Source: CAD feature listing. Evaluate the final solid. Frame: model axes, mm. A direction names the side the tool comes from. Give positions to 0.01 mm unless a question says otherwise; leave off trailing zeros. Order: outer loops, then holes, each group sorted by start corner. A loop starts at its lowest first (then second) coordinate and runs counter-clockwise, first axis right, second up. Notation, with made-up numbers: (-13, 39.5) - (6, 39.5) arc R20 ccw to (6, 77.5) - close; hole circle Ø3 at (35.25, 34.5). An arc over 180 degrees is marked (long way). Answer as CSV lines item,"result".
Autodesk Inventor part; units mm, degrees
ref_plane "YZ Plane" through (0, 0, 0) normal (1, 0, 0) x (0, 1, 0)
ref_plane "XZ Plane" through (0, 0, 0) normal (0, 1, 0) x (-1, 0, 0)
ref_plane "XY Plane" through (0, 0, 0) normal (0, 0, 1) x (1, 0, 0)
sketch "Skizze1" plane through (0, 0, 0) normal (0, 0, 1) x (1, 0, 0)
  line L0 (-5.275, 5.275) -> (5.275, 5.275)
  line L1 (5.275, 5.275) -> (5.275, -5.275)
  line L2 (5.275, -5.275) -> (-5.275, -5.275)
  line L3 (-5.275, -5.275) -> (-5.275, 5.275)
  line L4 (-5.275, 5.275) -> (5.275, -5.275) construction
  line L5 (5.275, 5.275) -> (-5.275, -5.275) construction
  line L6 (8.275, 8.275) -> (-8.275, 8.275)
  line L7 (-8.275, 8.275) -> (-8.275, -8.275)
  line L8 (-8.275, -8.275) -> (8.275, -8.275)
  line L9 (8.275, -8.275) -> (8.275, 8.275)
  point P0 (0, 0)
  dimension "d0" = 10.55
  dimension "d1" = 10.55
  dimension "d2" = 3
extrude "Extrusion1" add sketch "Skizze1" along normal blind 15
sketch "Skizze2" plane through (8.275, -8.275, 0) normal (1, 0, 0) x (0, 0, -1)
  line L0 (0, 0) -> (0, 16.55)
  line L1 (0, 16.55) -> (-15, 16.55)
  line L2 (-15, 0) -> (-15, 16.55)
  line L3 (0, 0) -> (-15, 0)
  circle A0 centre (-7.5, 22) radius 2.1
  circle A1 centre (-7.5, 22) radius 5.3
  line L4 (-15, 16.55) -> (-12.8, 22)
  line L5 (0, 16.55) -> (0, 0)
  line L6 (0, 16.55) -> (-2.2, 22)
  point P0 (0, 8.275)
  dimension "d5" = 4.2
  dimension "d6" = 22
  dimension "d7" = 7.5
  dimension "d8" = 3.2
extrude "Extrusion2" add sketch "Skizze2" against normal up to surface (16.55 mm away) contours L1 L4 A1 L6 | A1
fillet "Rundung1" radius 15.75 4 edges at (0, 13.725, 2.2) (0, 8.275, 0) (0, 8.275, 15) (0, 13.725, 12.8)
equation "\"d1\" = d0"
properties part number "AL_PipeMount"
(1) Access query for faces 1 (the flat face through (-5.275, 0, 7)), 2 (the cylindrical face through (0.116, 13.251, 13.067)). Directions: +Z, -Z, +X, -X, +Y, -Y. A direction counts if a zero-diameter tool reaches every point of the face in a straight line with its end or side. Return the directions, or none.
Completed:
face 1,"+Z, -Z"
face 2,"+Z, +X, -X, +Y"
(2) Mould query, pull axis X, two halves, no side actions, for faces 3 (the cylindrical face through (0.1, 13.8, 9.6)), 4 (the flat face through (5.275, 0, 7)), 5 (the flat face through (8.275, 2, 7)). Classes: released by +X, released by -X, zero draft, split by the parting line, or undercut.
Completed:
face 3,"zero draft"
face 4,"undercut"
face 5,"released by +X"
(3) Cut plane D-D (z = 12.25). Return loops of the section in (x, y) (3 decimals), then the cut area to 3 significant figures.
Completed:
outline,"(-8.275, -8.275) - (8.275, -8.275) - (8.275, 16.076) - (-8.275, 16.076) - close; hole (-5.275, -5.275) - (5.275, -5.275) - (5.275, 5.275) - (-5.275, 5.275) - close"
area,"292 mm²"
(4) Cut plane A-A (z = 7.5). Return loops of the section in (x, y) (3 decimals), then the cut area to 3 significant figures.
Completed:
outline,"(-8.275, -8.275) - (8.275, -8.275) - (8.275, 11.625) - (-8.275, 11.625) - close; (-8.275, 15.825) - (8.275, 15.825) - (8.275, 19.025) - (-8.275, 19.025) - close; hole (-5.275, -5.275) - (5.275, -5.275) - (5.275, 5.275) - (-5.275, 5.275) - close"
area,"271 mm²"
(5) Ray query, line 1 (Y direction, x = -0.25, z = 7.5) (3 decimals); line 2 (X direction, y = 3.75, z = 13.75) (3 decimals); line 3 (Z direction, x = -3.5, y = 11). Return the intervals inside material, ascending. Write a range as from..to.
Completed:
line 1,"-8.275..-5.275, 5.275..11.625, 15.825..19.025"
line 2,"-8.275..-5.275, 5.275..8.275"
line 3,"1.1..13.9"
(6) Cut plane C-C (x = 0). Return loops of the section in (y, z) (3 decimals).
Completed:
outline,"(-8.275, 0) - (-5.275, 0) - (-5.275, 15) - (-8.275, 15) - close; (5.275, 0) arc R15.75 ccw to (11.112, 1.145) - (11.847, 1.442) arc R15.75 cw to (14.737, 2.297) arc R5.3 ccw to (14.737, 12.703) arc R15.75 cw to (11.847, 13.558) - (11.112, 13.855) arc R15.75 ccw to (5.275, 15) - close; hole circle Ø4.2 at (13.725, 7.5)"
(7) Cut plane B-B (y = 4.5). Return loops of the section in (x, z) (3 decimals), then the cut area to 3 significant figures.
Completed:
outline,"(-8.275, 0) - (-5.275, 0) - (-5.275, 15) - (-8.275, 15) - close; (5.275, 0) - (8.275, 0) - (8.275, 15) - (5.275, 15) - close"
area,"90.0 mm²"
(8) Contact query for flat-ended pins moving along their axis: pin 1 (2 mm diameter, centred on x = 6.5, y = 15.5, fed in from +Z); pin 2 (3.5 mm diameter, centred on y = 13.725, z = 7.5, fed in from +X). Output: stop coordinate, or through.
Completed:
pin 1,"z = 12.75"
pin 2,"through"
